Autodesk Inventor part; units mm, degrees
ref_plane "YZ Plane" through (0, 0, 0) normal (1, 0, 0) x (0, 1, 0)
ref_plane "XZ Plane" through (0, 0, 0) normal (0, 1, 0) x (-1, 0, 0)
ref_plane "XY Plane" through (0, 0, 0) normal (0, 0, 1) x (1, 0, 0)
sketch "Skizze1" plane through (0, 0, 0) normal (0, 0, 1) x (1, 0, 0)
  line L0 (-17.5, -45) -> (17.5, -45)
  line L1 (17.5, -45) -> (17.5, 45)
  line L2 (17.5, 45) -> (-17.5, 45)
  line L3 (-17.5, 45) -> (-17.5, -45)
  line L4 (-17.5, -45) -> (17.5, 45) construction
  line L5 (17.5, -45) -> (-17.5, 45) construction
  point P0 (0, 0)
  dimension "d0" = 35
  dimension "d1" = 90
extrude "Extrusion1" add sketch "Skizze1" along normal blind 10
sketch "Skizze2" plane through (0, 0, 10) normal (0, 0, 1) x (1, 0, 0)
  line L0 (-17.5, -45) -> (17.5, -45)
  line L1 (17.5, -45) -> (17.5, 45)
  line L2 (-17.5, -45) -> (17.5, -45)
  line L3 (17.5, -45) -> (17.5, -35)
  line L4 (17.5, -35) -> (-17.5, -35)
  line L5 (-17.5, -35) -> (-17.5, -45)
  point P0 (0, 0)
  dimension "d4" = 10
extrude "Extrusion2" add sketch "Skizze2" along normal blind 30
sketch "Skizze3" plane through (0, 0, 0) normal (0, 0, -1) x (-1, 0, 0)
  line L0 (17.5, -45) -> (-17.5, -45)
  line L1 (-17.5, -45) -> (-17.5, -35)
  line L2 (-17.5, -35) -> (17.5, -35)
  line L3 (17.5, -35) -> (17.5, -45)
  line L4 (0, -63) -> (0, 63)
  line L5 (-17.5, -45) -> (-17.5, 45)
  line L6 (-17.5, -40) -> (17.5, -40)
  point P0 (0, 0)
  point P1 (0, 10)
  dimension "d7" = 50
hole "Bohrung1" at (0, 10, 0) direction (0, 0, 1) diameter 5.5 end through all counterbore diameter 10 counterbore depth 2.5
sketch "Skizze4" plane through (0, 0, 40) normal (0, 0, 1) x (1, 0, 0)
  line L0 (-17.5, -45) -> (17.5, -45)
  line L1 (17.5, -45) -> (17.5, -35)
  line L2 (17.5, -35) -> (-17.5, -35)
  line L3 (-17.5, -35) -> (-17.5, -45)
  line L4 (-17.5, -35) -> (17.5, -45) construction
  line L5 (-17.5, -35) -> (17.5, -35) construction
  line L6 (17.5, -35) -> (-17.5, -45) construction
  point P0 (0, 0)
  point P1 (0, -40)
hole "Bohrung2" at (0, -40, 40) direction (0, 0, -1) diameter 2.9 end through all
sketch "Skizze5" plane through (0, 0, 0) normal (1, 0, 0) x (0, 1, 0)
  line L0 (7.25, 10) -> (12.75, 10)
  line L1 (7.25, 2.5) -> (12.75, 2.5)
  line L2 (45, 10) -> (-35, 10)
  line L3 (-35, 10) -> (-35, 40)
  line L4 (-35, 40) -> (-4.9612, 10)
  line L5 (10.0388, 10) -> (10.0388, -4.326) construction
  line L6 (-35, 40) -> (-35, 10)
  line L7 (-4.9612, 10) -> (-35, 10)
  point P0 (0, 0)
  dimension "d22" = 15
extrude "Extrusion3" add sketch "Skizze5" along normal mid plane 10
properties part number "Verstrebung"
Read the model definition and answer for the solid it produces. Units are mm, in the model's axes. A direction names the side the tool comes from. Coordinates: 2 decimals unless noted, no trailing zeros. Write each loop counter-clockwise with the first axis right and the second up, starting at its lowest first coordinate (ties: lowest second). Pieces come first, ordered by that corner, then holes. Notation, with made-up numbers: (-13, 84) - (43, 84) arc R19 ccw to (43, 102) - close; hole circle Ø10 at (7.25, -15.75). An arc over 180 degrees is marked (long way). Answer as a JSON object with one key per item and string values. Group by question number.
1. The mould has two halves that part along Y. Classify faces 6 (the cylindrical face through (-0.06, -38.55, 19.72)), 7 (the flat face through (-5, -27, 19)), 8 (the flat face through (-11, -35, 25)): +Y half, -Y half, draft (parallel to the pull), parting line (faces both ways), or undercut.
2. Each of these flat-tipped pins is pushed along its axis until it touches: P1, Ø4, axis at x = -6, y = 0.5, coming from the -Z side; P2, Ø15, axis at y = -25, z = 25, coming from the -X side; P3, Ø7, axis at x = 0, y = 10, coming from the +Z side; P4, Ø4, axis at x = -12, z = 23.5, coming from the +Y side. Where does it stop, or does it pass through?
3. Which of the six approach directions +Z, -Z, +X, -X, +Y, -Y give full straight-line access (tool end or side, diameter ignored) to faces 1 (the flat face through (17.5, -10.2, 9.5)), 2 (the flat face through (0, 6, 10)), 3 (the cylindrical face through (-1.5, 14.77, 1.27)), 4 (the flat face through (5, -27, 19)), 5 (the flat face through (-0.07, -20.19, 25.21))?
4. A cutting plane is placed at D-D (y = 10). Determine the outline of the cut face in (x, z).
5. A cutting plane is placed at B-B (y = -40). Determine the outline of the cut face in (x, z), plus the area to 3 significant figures.
6. A cutting plane is placed at C-C (z = 11). Determine the outline of the cut face in (x, y), plus the area to 3 significant figures.
7. Consider L1, parallel to Y at x = 0, z = 7.5; L2, parallel to Y at x = 0, z = 1; L3, parallel to X at y = 10, z = 1.45. Determine where each line is inside the solid, lowest interval first. Write a range as [from, to].
8. A cutting plane is placed at A-A (x = 0). Determine the outline of the cut face in (y, z).
Worked out:
{
 "1": {"face 6": "undercut", "face 7": "draft", "face 8": "+Y half"},
 "2": {"P1": "stops at z = 0", "P2": "stops at x = -5", "P3": "stops at z = 10", "P4": "stops at y = -35"},
 "3": {"face 1": "+Z, -Z, +X, +Y, -Y", "face 2": "+Z, +Y", "face 3": "-Z", "face 4": "+Z, +X, +Y", "face 5": "+Z, +X, -X, +Y"},
 "4": {"outline": "(-17.5, 0) - (-5, 0) - (-5, 2.5) - (-2.75, 2.5) - (-2.75, 10) - (-17.5, 10) - close; (2.75, 2.5) - (5, 2.5) - (5, 0) - (17.5, 0) - (17.5, 10) - (2.75, 10) - close"},
 "5": {"outline": "(-17.5, 0) - (-1.45, 0) - (-1.45, 40) - (-17.5, 40) - close; (1.45, 0) - (17.5, 0) - (17.5, 40) - (1.45, 40) - close", "area": "1,280 mm²"},
 "6": {"outline": "(-17.5, -45) - (17.5, -45) - (17.5, -35) - (5, -35) - (5, -5.96) - (-5, -5.96) - (-5, -35) - (-17.5, -35) - close; hole circle Ø2.9 at (0, -40)", "area": "634 mm²"},
 "7": {"L1": "y = [-45, -41.45], [-38.55, 7.25], [12.75, 45]", "L2": "y = [-45, -41.45], [-38.55, 5], [15, 45]", "L3": "x = [-17.5, -5], [5, 17.5]"},
 "8": {"outline": "(-45, 0) - (-41.45, 0) - (-41.45, 40) - (-45, 40) - close; (-38.55, 0) - (5, 0) - (5, 2.5) - (7.25, 2.5) - (7.25, 10) - (-4.96, 10) - (-35, 40) - (-38.55, 40) - close; (12.75, 2.5) - (15, 2.5) - (15, 0) - (45, 0) - (45, 10) - (12.75, 10) - close"}
}
